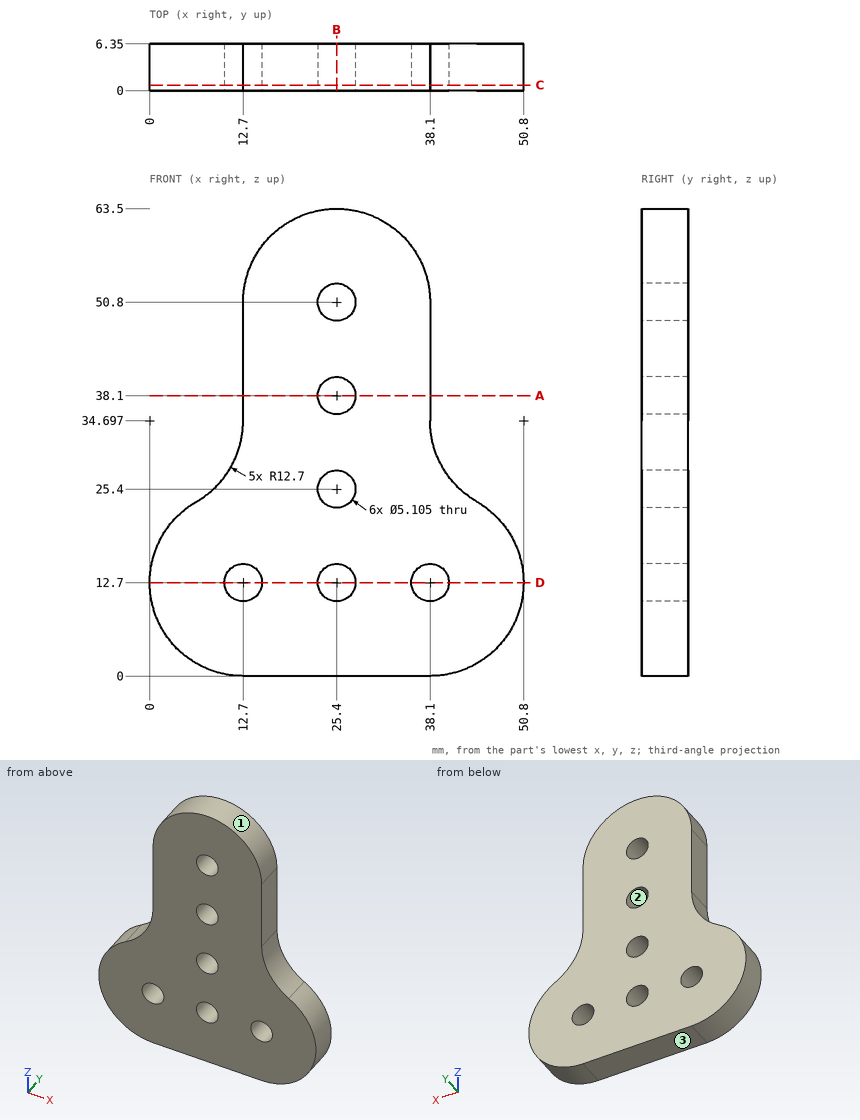
Job drawing, mm, ordinate dimensions from the low corner. One solid piece. Round coordinates to 2 decimals unless told otherwise and drop trailing zeros. Order: outer loops, then holes, each group sorted by start corner. A loop starts at its lowest first (then second) coordinate and runs counter-clockwise, first axis right, second up. Notation, with made-up numbers: (-21, 64) - (-6, 64) arc R19 cw to (-6, 84) - close; hole circle Ø3 at (12, -30.5). An arc over 180 degrees is marked (long way). Use CSV: the item, a comma, the result in double quotes. Start each with the question number.
1) Saw through at A-A (z = 38.1). List the corners of the cut face in (x, y), and give its area (3 significant figures).
2) Saw through at B-B (x = 25.4). List the corners of the cut face in (y, z).
3) Two-plate mould, pull along Z, no slides. Class the marked faces 1, 2 and 3: pulls with the +Z half, pulls with the -Z half, needs draft (parallel to the pull), parting line crosses it, or undercut.
4) Wall check: L1, parallel to X at y = 2, z = 12.7; L2, parallel to Z at x = 26, y = 1.5 (1 decimal); L3, parallel to X at y = 3, z = 27. Give the ranges that are in metal, low to high. Write a range as [from, to].
5) Pin check, flat tips, straight feed: pin 1 Ø3 at (y, z) = (3.5, 39.5) entering from +X; pin 2 Ø6.5 at (x, z) = (25.4, 50.8) entering from -Y; pin 3 Ø1 at (y, z) = (2.5, 9) entering from -X; pin 4 Ø3 at (y, z) = (3.5, 45) entering from -X. Stop position of each tip, or through.
6) Saw through at D-D (z = 12.7). List the corners of the cut face in (x, y).
7) Saw through at C-C (y = 0.75). Count the separate pieces of the cut face and the enclosed holes in it, and give its area (3 significant figures).
Values follow:
1,outline,"(12.7, 0) - (22.85, 0) - (22.85, 6.35) - (12.7, 6.35) - close; (27.95, 0) - (38.1, 0) - (38.1, 6.35) - (27.95, 6.35) - close"
1,area,"129 mm2"
2,outline,"(0, 0) - (6.35, 0) - (6.35, 10.15) - (0, 10.15) - close; (0, 15.25) - (6.35, 15.25) - (6.35, 22.85) - (0, 22.85) - close; (0, 27.95) - (6.35, 27.95) - (6.35, 35.55) - (0, 35.55) - close; (0, 40.65) - (6.35, 40.65) - (6.35, 48.25) - (0, 48.25) - close; (0, 53.35) - (6.35, 53.35) - (6.35, 63.5) - (0, 63.5) - close"
3,face 1,"pulls with the +Z half"
3,face 2,"undercut"
3,face 3,"pulls with the -Z half"
4,L1,"x = [0, 10.15], [15.25, 22.85], [27.95, 35.55], [40.65, 50.8]"
4,L2,"z = [0, 10.2], [15.2, 22.9], [27.9, 35.6], [40.6, 48.3], [53.3, 63.5]"
4,L3,"x = [10.1, 23.41], [27.39, 40.7]"
5,pin 1,"stops at x = 38.1"
5,pin 2,"stops at y = 0"
5,pin 3,"stops at x = 0.41"
5,pin 4,"stops at x = 12.7"
6,outline,"(0, 0) - (10.15, 0) - (10.15, 6.35) - (0, 6.35) - close; (15.25, 0) - (22.85, 0) - (22.85, 6.35) - (15.25, 6.35) - close; (27.95, 0) - (35.55, 0) - (35.55, 6.35) - (27.95, 6.35) - close; (40.65, 0) - (50.8, 0) - (50.8, 6.35) - (40.65, 6.35) - close"
7,separate pieces,"1"
7,enclosed holes,"6"
7,area,"1,950 mm2"
